For this review, take the finished solid that the model builds, in its own axes (mm). Face numbers are marked on the shaded views. A direction names the side the tool comes from. Give positions to 0.01 mm unless a question says otherwise; leave off trailing zeros. Write each loop counter-clockwise with the first axis right and the second up, starting at its lowest first coordinate (ties: lowest second). Pieces come first, ordered by that corner, then holes. Notation, with made-up numbers: M 61,-11.5 L 114,-11.5 A28 ccw 114,21.5 Z; hole C 27.25,41 d11. An arc over 180 degrees is marked long. One line per item, written item: value. Start each with the question number.
Item 1: Clearance check with flat-ended pins moving along their axes: pin 1 Ø2.5 at (x, y) = (31.5, -51) entering from +Z; pin 2 Ø2.5 at (x, y) = (27.5, 49) entering from -Z; pin 3 Ø9.5 at (x, y) = (30.5, -49) entering from -Z. State where each tip first meets the part, or that it passes through.
Item 2: Consider section B-B, the plane y = -49. Write out the cut boundary in (x, z).
Item 3: Consider section C-C, the plane x = 20. Write out the cut boundary in (y, z) (3 decimals), and give its area (3 significant figures).
Item 4: To check wall thickness, follow probe 1 along Y at (x, z) = (27.75, 0); probe 2 along Z at (x, y) = (17.5, 54.5); probe 3 along X at (y, z) = (-13, 30). State the ranges of each line that lie inside material, in increasing order.
Item 5: Mouldability with a two-part tool opening along Z and no side actions: class the marked faces 4, 5, 6 and 7 as released by +Z, released by -Z, zero draft, split by the parting line, or undercut.
Item 6: Consider section D-D, the plane y = 0. Write out the cut boundary in (x, z) (3 decimals), and give its area (3 significant figures).
Item 7: Tool access review of the marked faces 1, 2 and 3: name each direction out of +Z, -Z, +X, -X, +Y, -Y from which nothing blocks a thin tool from reaching the whole face with its end or side.
Item 8: Consider section A-A, the plane z = 0. Write out the cut boundary in (x, y) (3 decimals), and give its area (3 significant figures).
```python
from build123d import *

# Parameters (mm, degrees)
SKETCH1_W           = 17.145
SKETCH1_H           = 18.25
SKETCH2_R           = 3.71475
CUT_EXTRUDE1_DEPTH  = 8.5725
SKETCH3_R           = 18.25
BOSS_EXTRUDE1_DEPTH = 8.5
SKETCH4_R           = 4.45
BOSS_EXTRUDE2_DEPTH = 46
SKETCH5_R           = 18.25
CUT_EXTRUDE2_DEPTH  = 22.15


with BuildPart() as part:
    # Sketch1 → Revolve1 (revolve)
    with BuildSketch(Plane.XY):
        with Locations((16.8275, 9.125)):
            Rectangle(SKETCH1_W, SKETCH1_H)
    revolve(axis=Axis((8.255, 0, 0), (1, 0, 0)))

    # Sketch2 → Cut-Extrude1 (cut)
    with BuildSketch(Plane.ZY.offset(-8.255)):
        Circle(SKETCH2_R)
    extrude(amount=-CUT_EXTRUDE1_DEPTH, mode=Mode.SUBTRACT)


with BuildPart() as body_2:
    # Sketch3 → Boss-Extrude1 (new body)
    with BuildSketch(Plane(origin=(25.4, 0, 0), x_dir=(0, 0, -1), z_dir=(1, 0, 0))):
        with BuildLine():
            Line((-24.382347836, 32.115154563), (-32.324530318, 17.115154563))
            ThreePointArc((-32.324530318, 17.115154563), (-36.576, 0), (-32.324530318, -17.115154563))
            Line((-32.324530318, -17.115154563), (-24.382347836, -32.115154563))
            ThreePointArc((-24.382347836, -32.115154563), (-21.780072988, -38.920854003), (-20.89525, -46.153175037))
            Line((-20.89525, -46.153175037), (-20.89525, -55))
            ThreePointArc((-20.89525, -55), (-13.175, -62.72025), (-5.45475, -55))
            Line((-5.45475, -55), (-5.45475, -44))
            ThreePointArc((-5.45475, -44), (0, -38.54525), (5.45475, -44))
            Line((5.45475, -44), (5.45475, -55))
            ThreePointArc((5.45475, -55), (13.175, -62.72025), (20.89525, -55))
            Line((20.89525, -55), (20.89525, -46.153175037))
            ThreePointArc((20.89525, -46.153175037), (21.780072988, -38.920854003), (24.382347836, -32.115154563))
            Line((24.382347836, -32.115154563), (32.324530318, -17.115154563))
            ThreePointArc((32.324530318, -17.115154563), (36.576, 0), (32.324530318, 17.115154563))
            Line((32.324530318, 17.115154563), (24.382347836, 32.115154563))
            ThreePointArc((24.382347836, 32.115154563), (21.780072988, 38.920854003), (20.89525, 46.153175037))
            Line((20.89525, 46.153175037), (20.89525, 55))
            ThreePointArc((20.89525, 55), (13.175, 62.72025), (5.45475, 55))
            Line((5.45475, 55), (5.45475, 44))
            ThreePointArc((5.45475, 44), (0, 38.54525), (-5.45475, 44))
            Line((-5.45475, 44), (-5.45475, 55))
            ThreePointArc((-5.45475, 55), (-13.175, 62.72025), (-20.89525, 55))
            Line((-20.89525, 55), (-20.89525, 46.153175037))
            ThreePointArc((-20.89525, 46.153175037), (-21.780072988, 38.920854003), (-24.382347836, 32.115154563))
        make_face()
        Circle(SKETCH3_R, mode=Mode.SUBTRACT)
        Circle(SKETCH3_R)
    extrude(amount=BOSS_EXTRUDE1_DEPTH)

    # Sketch4 → Boss-Extrude2 (add)
    with BuildSketch(Plane.ZY.offset(-25.4)):
        with Locations((-13.175, 55)):
            Circle(SKETCH4_R)
        with Locations((13.175, -55)):
            Circle(SKETCH4_R)
        with Locations((13.175, 55)):
            Circle(SKETCH4_R)
        with Locations((-13.175, -55)):
            Circle(SKETCH4_R)
    extrude(amount=BOSS_EXTRUDE2_DEPTH)


with BuildPart() as cut_extrude2_tool:
    # Sketch5 → Cut-Extrude2 (new body)
    with BuildSketch(Plane.ZY.offset(-8.255)):
        Circle(SKETCH5_R)
    extrude(amount=-CUT_EXTRUDE2_DEPTH)


with BuildPart() as part_1:
    add(part.part)

    # Cut-Extrude2: cut by cut_extrude2_tool
    add(cut_extrude2_tool.part, mode=Mode.SUBTRACT)


with BuildPart() as body_2_1:
    add(body_2.part)

    # Cut-Extrude2: cut by cut_extrude2_tool
    add(cut_extrude2_tool.part, mode=Mode.SUBTRACT)


solid = body_2_1.part
```
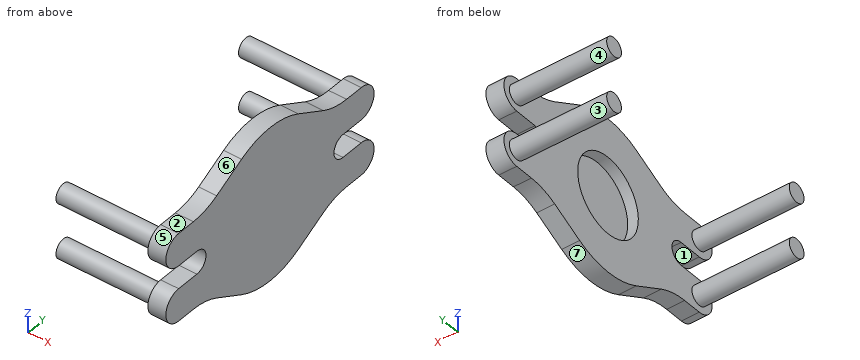
Model answer:
1. pin 1: stops at z = 20.9
1. pin 2: stops at z = -20.9
1. pin 3: stops at z = -20.96
2. outline: M 25.4,-20.9 L 33.9,-20.9 L 33.9,-5.45 L 25.4,-5.45 Z; M 25.4,5.45 L 33.9,5.45 L 33.9,20.9 L 25.4,20.9 Z
3. outline: C -55,-13.175 d8.9; C -55,13.175 d8.9; C 55,-13.175 d8.9; C 55,13.175 d8.9
3. area: 249 mm2
4. probe 1: y = -38.55 to -18.25, 18.25 to 38.55
4. probe 2: z = -17.6 to -8.75, 8.75 to 17.6
4. probe 3: x = 25.4 to 33.9
5. face 4: undercut
5. face 5: undercut
5. face 6: released by +Z
5. face 7: released by -Z
6. outline: M 25.4,-36.576 L 33.9,-36.576 L 33.9,36.576 L 25.4,36.576 L 25.4,18.25 L 30.405,18.25 L 30.405,-18.25 L 25.4,-18.25 Z
6. area: 439 mm2
7. face 1: +X, -X, -Y
7. face 2: +Z, +X, -X, -Y
7. face 3: -X
8. outline: M 25.4,-38.545 L 33.9,-38.545 L 33.9,38.545 L 25.4,38.545 L 25.4,18.25 L 30.405,18.25 L 30.405,-18.25 L 25.4,-18.25 Z
8. area: 473 mm2
